Can you work these out from the model? Positions are in its coordinate system, mm. Face numbers are marked on the shaded views. A direction names the side the tool comes from. Round coordinates to 2 decimals unless told otherwise and drop trailing zeros. Loops run counter-clockwise (first coordinate to the right, second up) from the corner with the lowest first, then second, coordinate; pieces in that order, holes last. Notation, with made-up numbers: (56.5, 3) -> (64.5, 3) arc R13 cw to (64.5, 13) -> close; hole circle Ø9 at (30.25, 7.5). An arc over 180 degrees is marked (long way). Write item = value, one per line.
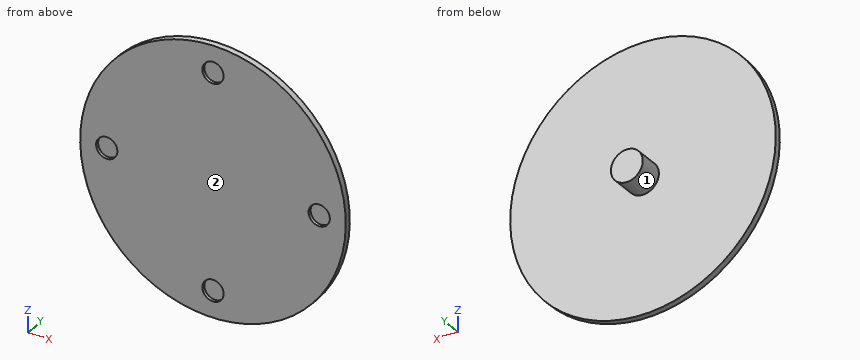
from build123d import *

# Parameters (mm, degrees)
SKETCH1_R                               = 125
SKETCH1_R_2                             = 10
BOSS_EXTRUDE1_DEPTH                     = 3
SKETCH2_R                               = 125
B_T_CH_N_DRONE_DEPTH                    = 3
SKETCH3_R                               = 15
TR_C_G_N_V_O_V_NG_BI_THAY_I_MATCH_DEPTH = 24


with BuildPart() as part:
    # Sketch1 → Boss-Extrude1 (new body)
    with BuildSketch(Plane(origin=(0, 0, 0), x_dir=(1, 0, 0), z_dir=(0, 1, 0))):
        with Locations(Location((0, 0, 0), (0, 0, 270))):
            Circle(SKETCH1_R)
        with Locations(Location((0, 100, 0), (0, 0, 270))):
            Circle(SKETCH1_R_2, mode=Mode.SUBTRACT)
        with Locations(Location((100, 0, 0), (0, 0, 270))):
            Circle(SKETCH1_R_2, mode=Mode.SUBTRACT)
        with Locations(Location((0, -100, 0), (0, 0, 270))):
            Circle(SKETCH1_R_2, mode=Mode.SUBTRACT)
        with Locations(Location((-100, 0, 0), (0, 0, 270))):
            Circle(SKETCH1_R_2, mode=Mode.SUBTRACT)
    extrude(amount=BOSS_EXTRUDE1_DEPTH)

    # Sketch2 → bắt chân drone (add)
    with BuildSketch(Plane(origin=(0, 3, 0), x_dir=(1, 0, 0), z_dir=(0, 1, 0))):
        with Locations(Location((0, 0, 0), (0, 0, 270))):
            Circle(SKETCH2_R)
    extrude(amount=B_T_CH_N_DRONE_DEPTH)

    # Sketch3 → Trục gắn vào vòng bi (Thay đổi để match) (add)
    with BuildSketch(Plane(origin=(0, 6, 0), x_dir=(1, 0, 0), z_dir=(0, 1, 0))):
        with Locations(Location((0, 0, 0), (0, 0, 270))):
            Circle(SKETCH3_R)
    extrude(amount=TR_C_G_N_V_O_V_NG_BI_THAY_I_MATCH_DEPTH)


solid = part.part
1. Suppose I cut it at A-A, the plane z = -100. List the corners of the cut face in (x, y) for me, and give its area (3 significant figures).
Entries:
outline = (-75, 0) -> (-10, 0) -> (-10, 3) -> (10, 3) -> (10, 0) -> (75, 0) -> (75, 6) -> (-75, 6) -> close
area = 840 mm²
2. I need wall thicknesses on line 1 (X direction, y = 1.6, z = 0); line 2 (Y direction, x = 22, z = -80.5); line 3 (X direction, y = 0.7, z = 100). Which ranges of each line are inside material? Lowest first, please. Write a range as [from, to].
Entries:
line_1 = [-125, -110], [-90, 90], [110, 125]
line_2 = [0, 6]
line_3 = [-75, -10], [10, 75]
3. Suppose I cut it at B-B, the plane x = 100. List the corners of the cut face in (y, z) for me, and give its area (3 significant figures).
Entries:
outline = (0, -75) -> (6, -75) -> (6, 75) -> (0, 75) -> (0, 10) -> (3, 10) -> (3, -10) -> (0, -10) -> close
area = 840 mm²
4. Suppose I cut it at D-D, the plane y = 10.25. List the corners of the cut face in (x, z) for me.
Entries:
outline = circle Ø30 at (0, 0)
5. I'm going to push flat-ended pins straight in: pin 1 (3 mm diameter, centred on y = 25, z = -14, fed in from -X); pin 2 (16 mm diameter, centred on x = 0, z = -100, fed in from -Y); pin 3 (3 mm diameter, centred on x = 4, z = -81, fed in from +Y). Where does each tip first touch, or does it pass through?
Entries:
pin_1 = -8.29
pin_2 = 3
pin_3 = 6
6. Suppose I cut it at C-C, the plane x = 0. List the corners of the cut face in (y, z) for me.
Entries:
outline = (0, -125) -> (6, -125) -> (6, -15) -> (30, -15) -> (30, 15) -> (6, 15) -> (6, 125) -> (0, 125) -> (0, 110) -> (3, 110) -> (3, 90) -> (0, 90) -> (0, -90) -> (3, -90) -> (3, -110) -> (0, -110) -> close
7. For the marked faces 1 and 2, which set-ups out of +Z, -Z, +X, -X, +Y, -Y let a thin tool reach every point of the face, with its end or its side?
Entries:
face_1 = +Y
face_2 = +Z, -Z, +X, -X, -Y
